from build123d import *

# Parameters (mm, degrees)
F2_R     = 2.921
F3_DEPTH = 19.05
F5_R     = 2.2225
F6_DEPTH = 3.175


with BuildPart() as f1:
    # F0 (on Front) → F1 (revolve)
    with BuildSketch(Plane.XZ):
        with BuildLine():
            Line((0, 0), (0, -12.7))
            ThreePointArc((0, -12.7), (12.7, 0), (0, 12.7))
            Line((0, 12.7), (0, 0))
        make_face()
    revolve(axis=Axis((0, 0, 6.35), (0, 0, 1)))

    # F2 (on Top) → F3 (join)
    with BuildSketch(Plane.XY):
        Circle(F2_R)
    extrude(amount=-F3_DEPTH)

    # F5 (on offset) → F6 (cut)
    with BuildSketch(Plane.XZ.offset(12.7)):
        with Locations((-3.81, 4.271358)):
            Circle(F5_R)
        with Locations((3.81, 4.271358)):
            Circle(F5_R)
        with BuildLine():
            ThreePointArc((-4.331955, -2.855323), (-5.431521, -2.629416), (-5.657427, -3.728982))
            ThreePointArc((-5.657427, -3.728982), (0, -6.775824), (5.657427, -3.728982))
            ThreePointArc((5.657427, -3.728982), (5.431521, -2.629416), (4.331955, -2.855323))
            ThreePointArc((4.331955, -2.855323), (0, -5.188324), (-4.331955, -2.855323))
        make_face()
    extrude(amount=-F6_DEPTH, mode=Mode.SUBTRACT)


solid = f1.part
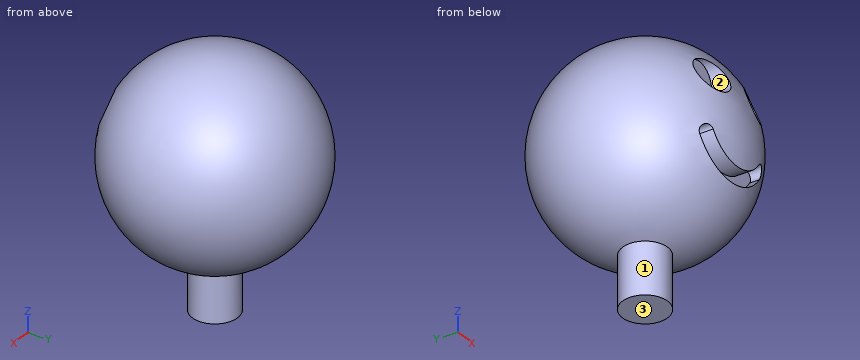
Work out the finished part from the listing and answer in its coordinate system (mm). Face numbers are marked on the shaded views. Round coordinates to 2 decimals unless told otherwise and drop trailing zeros. Order: outer loops, then holes, each group sorted by start corner. A loop starts at its lowest first (then second) coordinate and runs counter-clockwise, first axis right, second up. Notation, with made-up numbers: M 6.5,47 L 54.5,47 A10 ccw 54.5,60 Z; hole C -20.75,88 d8. An arc over 180 degrees is marked long. Put each result on its own line as item: value. Start each with the question number.
Q1. Section B-B, the plane z = 3 is taken. Write down the section's boundary in (x, y) (3 decimals).
Q2. Section D-D, the plane z = -15 is taken. Write down the section's boundary in (x, y).
Q3. Flat-ended cylindrical pins translate along their axes: pin 1 (8 mm diameter, centred on y = 8, z = -3, fed in from +X); pin 2 (10 mm diameter, centred on x = -8.5, z = -10, fed in from +Y); pin 3 (3.5 mm diameter, centred on x = -4, z = 4, fed in from -Y) (3 decimals); pin 4 (4 mm diameter, centred on x = 3.5, y = 3, fed in from -Z). Find the tip coordinate at first contact, or state that the pin passes through.
Q4. Straight lines are drawn through the part: L1, parallel to Z at x = 3.81, y = -10.05; L2, parallel to X at y = -9, z = 1; L3, parallel to Z at x = 3.81, y = -11.15. For each, find the intervals that lie inside material, in ascending order. Write a range as [from, to].
Q5. For a pull along X with two mould halves and no side action, classify the marked faces 1, 2 and 3 as pulls with the +X half, pulls with the -X half, needs draft (parallel to the pull), parting line crosses it, or undercut.
Q6. Section C-C, the plane y = -6.25 is taken. Write down the section's boundary in (x, z).
Q7. Section A-A, the plane x = 0 is taken. Write down the section's boundary in (y, z) (3 decimals).
Findings below:
1. outline: M -5.633,-10.98 L -5.633,-9.525 L -1.987,-9.525 L -1.987,-12.18 A12.341 ccw 1.987,-12.18 L 1.987,-9.525 L 5.633,-9.525 L 5.633,-10.98 A12.341 ccw long Z
2. outline: C 0,0 d5.84
3. pin 1: stops at x = 11.86
3. pin 2: stops at y = 9.76
3. pin 3: stops at y = -9.525
3. pin 4: stops at z = -19.05
4. L1: z = [-6.77, -5.6], [-3.52, 2.05], [6.49, 6.77]
4. L2: x = [-8.9, 8.9]
4. L3: z = [-3.52, 2.05]
5. face 1: parting line crosses it
5. face 2: undercut
5. face 3: needs draft
6. outline: C 0,0 d22.11
7. outline: M -11.592,-5.188 L -9.525,-5.188 L -9.525,-6.776 L -10.741,-6.776 A12.7 ccw -2.921,-12.36 L -2.921,-19.05 L 2.921,-19.05 L 2.921,-12.36 A12.7 ccw long Z
